Autodesk Inventor part; units mm, degrees
ref_plane "YZ Plane" through (0, 0, 0) normal (1, 0, 0) x (0, 1, 0)
ref_plane "XZ Plane" through (0, 0, 0) normal (0, 1, 0) x (-1, 0, 0)
ref_plane "XY Plane" through (0, 0, 0) normal (0, 0, 1) x (1, 0, 0)
sketch "Sketch1" plane through (0, 0, 0) normal (0, 0, 1) x (1, 0, 0)
  line L0 (-100, -15) -> (100, -15)
  line L1 (100, -15) -> (100, 15)
  line L2 (100, 15) -> (-100, 15)
  line L3 (-100, 15) -> (-100, -15)
  line L4 (-100, -15) -> (100, 15) construction
  line L5 (100, -15) -> (-100, 15) construction
  line L6 (-79.5, 20) -> (79.5, 20)
  line L7 (79.5, 20) -> (79.5, 15)
  line L8 (79.5, 15) -> (-79.5, 15)
  line L9 (-79.5, 15) -> (-79.5, 20)
  line L10 (-79.5, 20) -> (79.5, 15) construction
  line L11 (79.5, 20) -> (-79.5, 15) construction
  line L12 (-100, 0) -> (100, 0)
  line L13 (-79.5, -20) -> (79.5, -20)
  line L14 (79.5, -20) -> (79.5, -15)
  line L15 (79.5, -15) -> (-79.5, -15)
  line L16 (-79.5, -15) -> (-79.5, -20)
  line L17 (-79.5, -20) -> (79.5, -15) construction
  line L18 (79.5, -20) -> (-79.5, -15) construction
  point P0 (0, 0)
  point P1 (0, 17.5)
  point P2 (0, 15)
  point P3 (0, -17.5)
  point P4 (0, -15)
  dimension "d0" = 5
  dimension "d1" = 30
  dimension "d2" = 200
  dimension "d3" = 159
extrude "Plate1" add sketch "Sketch1" along normal blind 5
equation "\"d4\" = Thickness"
equation "\"BendRadius\" = Thickness"
equation "\"BendReliefWidth\" = Thickness"
equation "\"BendReliefDepth\" = 0.5 * Thickness"
equation "\"TransitionRadius\" = BendRadius"
equation "\"JacobiRadiusSize\" = BendRadius"
equation "\"GapSize\" = Thickness"
properties part number "Base Leg V1"
Geometry check sheet. Reference: the model listing, model coordinates, mm. A direction names the side the tool comes from. Give positions to 0.01 mm unless a question says otherwise; leave off trailing zeros. Loops run counter-clockwise (first coordinate to the right, second up) from the corner with the lowest first, then second, coordinate; pieces in that order, holes last. Notation, with made-up numbers: M 70,-35.5 L 82,-35.5 A26 cw 82,1.5 Z; hole C 75.25,16.25 d9. An arc over 180 degrees is marked long. Write item = value, one per line. Start each with the question number.
1. Thickness scan on probe 1 along Y at (x, z) = (-86.5, 4.7). Record the ranges inside material, lowest first.
2. Go/stop test with flat-tipped pins: P1, Ø2.5, axis at x = 86, z = 3, coming from the -Y side; P2, Ø6, axis at x = -7.5, y = -2.5, coming from the -Z side; P3, Ø2.5, axis at x = 84.5, z = 2.5, coming from the +Y side; P4, Ø2.5, axis at y = 16.5, z = 2, coming from the -X side. Record where each tip stops, or that it passes through.
3. Section check B-B, the plane x = 85. Enter the section's corners in (y, z).
4. Section check A-A, the plane z = 3.35. Enter the section's corners in (x, y).
5. Tool access check on faces 1 (the face through (-79.5, 17, 2)), 2 (the face through (-1, 20, 2)), 3 (the face through (-90, -15, 2)), 4 (the face through (90, -15, 2)), 5 (the face through (79.5, 18, 2)). Record the directions out of +Z, -Z, +X, -X, +Y, -Y that give a thin tool (end or side, any length) a straight path to the whole face; none if there is none.
Values follow:
q1.probe_1 = -15 to 15
q2.P1 = -15
q2.P2 = 0
q2.P3 = 15
q2.P4 = -79.5
q3.outline = M -15,0 L 15,0 L 15,5 L -15,5 Z
q4.outline = M -100,-15 L -79.5,-15 L -79.5,-20 L 79.5,-20 L 79.5,-15 L 100,-15 L 100,15 L 79.5,15 L 79.5,20 L -79.5,20 L -79.5,15 L -100,15 Z
q5.face_1 = +Z, -Z, -X, +Y
q5.face_2 = +Z, -Z, +X, -X, +Y
q5.face_3 = +Z, -Z, -X, -Y
q5.face_4 = +Z, -Z, +X, -Y
q5.face_5 = +Z, -Z, +X, +Y
